Answer from the drawing. Dimensions are ordinates in mm from the lowest x, y and z of the part. Round coordinates to 2 decimals unless told otherwise and drop trailing zeros. Loops run counter-clockwise (first coordinate to the right, second up) from the corner with the lowest first, then second, coordinate; pieces in that order, holes last. Notation, with made-up numbers: M -29,-38.75 L 4,-38.75 A23 ccw 4,0.25 Z; hole C 80.25,-36.75 d4. An arc over 180 degrees is marked long. Answer as CSV lines item,"result".
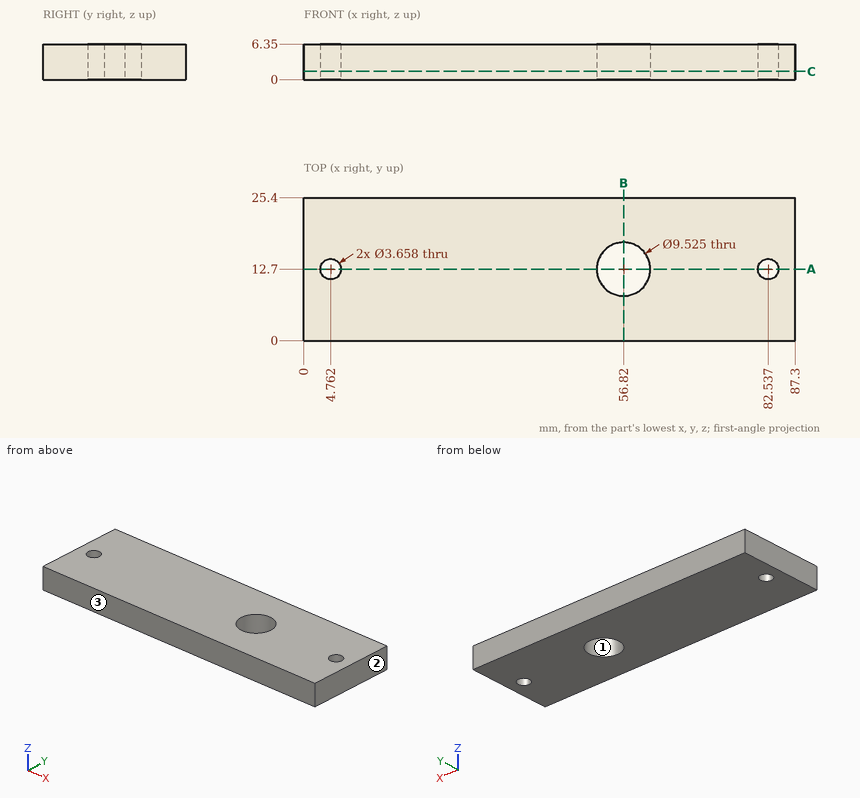
1) Determine the mould class of the marked faces 1, 2 and 3 for opening direction Y: released by +Y, released by -Y, zero draft, split by the parting line, or undercut.
Evaluation:
face 1,"undercut"
face 2,"zero draft"
face 3,"released by -Y"
2) Find section C-C, the plane z = 1.5. Give the vertices of the cut face in (x, y) (1 decimal), then the cut area to 4 significant figures.
Evaluation:
outline,"M 0,0 L 87.3,0 L 87.3,25.4 L 0,25.4 Z; hole C 4.8,12.7 d3.7; hole C 56.8,12.7 d9.5; hole C 82.5,12.7 d3.7"
area,"2,125 mm^2"
3) Find section B-B, the plane x = 56.82. Give the vertices of the cut face in (y, z), then the cut area to 3 significant figures.
Evaluation:
outline,"M 0,0 L 7.94,0 L 7.94,6.35 L 0,6.35 Z; M 17.46,0 L 25.4,0 L 25.4,6.35 L 17.46,6.35 Z"
area,"101 mm^2"
4) Straight lines are drawn through the part: line 1 (Y direction, x = 82.5, z = 2.5); line 2 (X direction, y = 9, z = 3.75); line 3 (Y direction, x = 81.5, z = 0.75) (1 decimal). For each, find the intervals that lie inside material, in ascending order.
Evaluation:
line 1,"y = 0 to 10.87, 14.53 to 25.4"
line 2,"x = 0 to 53.82, 59.82 to 87.3"
line 3,"y = 0 to 11.2, 14.2 to 25.4"
5) Find section A-A, the plane y = 12.7. Give the vertices of the cut face in (x, z).
Evaluation:
outline,"M 0,0 L 2.93,0 L 2.93,6.35 L 0,6.35 Z; M 6.59,0 L 52.06,0 L 52.06,6.35 L 6.59,6.35 Z; M 61.58,0 L 80.71,0 L 80.71,6.35 L 61.58,6.35 Z; M 84.37,0 L 87.3,0 L 87.3,6.35 L 84.37,6.35 Z"
